from build123d import *

# Parameters (mm, degrees)
BOSS_EXTRU_1_DEPTH      = 6
ESQUISSE2_R             = 0.5
ESQUISSE2_R_2           = 2.5
ENL_V_MAT_EXTRU_1_DEPTH = 6


with BuildPart() as part:
    # Esquisse1 → Boss.-Extru.1 (new body)
    with BuildSketch(Plane(origin=(0, 0, 0), x_dir=(0, 0, -1), z_dir=(1, 0, 0))):
        with BuildLine():
            Line((90, -12.5), (-90, -12.5))
            ThreePointArc((-90, -12.5), (-97.071067812, -9.571067812), (-100, -2.5))
            Line((-100, -2.5), (-100, 2.5))
            ThreePointArc((-100, 2.5), (-97.071067812, 9.571067812), (-90, 12.5))
            Line((-90, 12.5), (90, 12.5))
            ThreePointArc((90, 12.5), (97.071067812, 9.571067812), (100, 2.5))
            Line((100, 2.5), (100, -2.5))
            ThreePointArc((100, -2.5), (97.071067812, -9.571067812), (90, -12.5))
        make_face()
    extrude(amount=BOSS_EXTRU_1_DEPTH)

    # Esquisse2 → Enlèv. mat.-Extru.1 (cut)
    with BuildSketch(Plane.ZY):
        with Locations((-97, 0)):
            Circle(ESQUISSE2_R)
        with Locations((-92, 5)):
            Circle(ESQUISSE2_R)
        with Locations(Location((-92, -5, 0), (0, 0, 180))):
            Circle(ESQUISSE2_R)
        with Locations(Location((-87, 0, 0), (0, 0, 180))):
            Circle(ESQUISSE2_R)
        with Locations((-50, 0)):
            Circle(ESQUISSE2_R_2)
        Circle(ESQUISSE2_R_2)
        with Locations((50, 0)):
            Circle(ESQUISSE2_R_2)
    extrude(amount=-ENL_V_MAT_EXTRU_1_DEPTH, mode=Mode.SUBTRACT)


solid = part.part
Check sheet for the modelled part. Datum: model origin and axes. Units: mm. Round coordinates to 2 decimals unless told otherwise and drop trailing zeros. Loops run counter-clockwise (first coordinate to the right, second up) from the corner with the lowest first, then second, coordinate; pieces in that order, holes last. Notation, with made-up numbers: (68, -0.5) -> (84, -0.5) arc R31 cw to (84, 34.5) -> close; hole circle Ø9 at (-11, 56). An arc over 180 degrees is marked (long way). Put each result on its own line as item: value. Start each with the question number.
1. Gauge pin test, flat end, axial feed: pin 1 (3 mm diameter, centred on x = 3.5, y = 5, fed in from -Z). Record the tip position at first contact, or that the pin passes through.
2. Scan lines: probe 1 along Y at (x, z) = (3.5, 50); probe 2 along Y at (x, z) = (2.75, -87); probe 3 along Y at (x, z) = (3.1, -92). Record each from-to range of solid material in increasing order.
3. Section check A-A (x = 1.05). Enter the section's corners in (y, z), plus the area to 3 significant figures.
4. Section check B-B (z = 50). Enter the section's corners in (x, y), plus the area to 3 significant figures.
5. Section check C-C (y = -9.25). Enter the section's corners in (x, z).
6. Draft check along Y on faces 1 (the face through (2.96, -0.96, -47.69)), 2 (the face through (2.96, -9.49, -97.15)), 3 (the face through (2.96, 9.49, 97.15)). Enter one of: +Y half, -Y half, draft (parallel to the pull), parting line (faces both ways), or undercut.
Findings:
1. pin 1: stops at z = -99.95
2. probe 1: y = -12.5 to -2.5, 2.5 to 12.5
2. probe 2: y = -12.5 to -0.5, 0.5 to 12.5
2. probe 3: y = -12.3 to -5.5, -4.5 to 4.5, 5.5 to 12.3
3. outline: (-12.5, -90) arc R10 ccw to (-2.5, -100) -> (2.5, -100) arc R10 ccw to (12.5, -90) -> (12.5, 90) arc R10 ccw to (2.5, 100) -> (-2.5, 100) arc R10 ccw to (-12.5, 90) -> close; hole circle Ø1 at (-5, -92); hole circle Ø5 at (0, -50); hole circle Ø5 at (0, 0); hole circle Ø5 at (0, 50); hole circle Ø1 at (0, -97); hole circle Ø1 at (0, -87); hole circle Ø1 at (5, -92)
3. area: 4,850 mm^2
4. outline: (0, -12.5) -> (6, -12.5) -> (6, -2.5) -> (0, -2.5) -> close; (0, 2.5) -> (6, 2.5) -> (6, 12.5) -> (0, 12.5) -> close
4. area: 120 mm^2
5. outline: (0, -97.38) -> (6, -97.38) -> (6, 97.38) -> (0, 97.38) -> close
6. face 1: undercut
6. face 2: -Y half
6. face 3: +Y half
